Can you work these out from the model? Positions are in its coordinate system, mm. A direction names the side the tool comes from. Coordinates: 2 decimals unless noted, no trailing zeros. Order: outer loops, then holes, each group sorted by start corner. A loop starts at its lowest first (then second) coordinate and runs counter-clockwise, first axis right, second up. Notation, with made-up numbers: (85, -17.5) - (106, -17.5) arc R22 ccw to (106, 15.5) - close; hole circle Ø3 at (27.25, 15). An arc over 180 degrees is marked (long way). Use a Markdown table: item, result. Add a question column.
(1) If I drill on L1, parallel to Y at x = 0, z = -7; L2, parallel to X at y = 1.15, z = -2.25; L3, parallel to X at y = 0, z = -7.3, over which ranges is the centre line in solid material (lowest first)? Write a range as [from, to].
(2) For pin 1 Ø1 at (x, y) = (-2.5, -0.5) entering from +Z; pin 2 Ø2 at (x, z) = (-2.5, -2) entering from +Y; pin 3 Ø1.6 at (x, y) = (-12.5, 0) entering from +Z; pin 4 Ø2.5 at (x, y) = (12, 0) entering from -Z, each with a flat end and sliding along its axis, tell me the tip position at first contact or that it passes through.
(3) I want a section at D-D (x = -8). List the corners of the cut face in (y, z) for me.
(4) I want a section at C-C (z = -7). List the corners of the cut face in (x, y) for me.
(5) I want a section at A-A (x = 12.5). List the corners of the cut face in (y, z) for me.
(6) We'd pull the mould along Z, two halves only. Please class faces 3 (the flat face through (-13, 0, -2)), 4 (the conical face through (-11.082, -0.588, -0.396)), 5 (the conical face through (13.918, -0.588, -0.396)), 6 (the flat face through (15, 0, -1)): pulls with the +Z half, pulls with the -Z half, needs draft (parallel to the pull), parting line crosses it, or undercut.
(7) On a 3-axis mill with a long thin cutter (end or side, diameter ignored), from which of +Z, -Z, +X, -X, +Y, -Y can I reach the whole of each face in a straight line? I mean faces 1 (the flat face through (12, 0, -2)), 2 (the flat face through (-10, 0, 0)). Say none if no direction works.
(8) I want a section at B-B (z = -4.25). List the corners of the cut face in (x, y) for me.
```python
from build123d import *

# Parameters (mm, degrees)
F1_DEPTH = 2.5
F3_R     = 1.5
F4_DEPTH = 1
F4_TAPER = -5
F5_DEPTH = 25


with BuildPart() as f1:
    # F0 (on Front) → F1 (new body, symmetric)
    with BuildSketch(Plane.XZ):
        with BuildLine():
            ThreePointArc((0, -5), (-3.5355339059, -3.5355339059), (-5, 0))
            Line((-5, 0), (-15, 0))
            Line((-15, 0), (-15, -2))
            Line((-15, -2), (-10, -2))
            Line((-10, -2), (-5, -10.6602540378))
            Line((-5, -10.6602540378), (0, -10.6602540378))
            Line((0, -10.6602540378), (5, -10.6602540378))
            Line((5, -10.6602540378), (10, -2))
            Line((10, -2), (15, -2))
            Line((15, -2), (15, 0))
            Line((15, 0), (5, 0))
            ThreePointArc((5, 0), (3.5355339059, -3.5355339059), (0, -5))
        make_face()
    extrude(amount=F1_DEPTH, both=True)

    # F3 (on offset) → F4 (cut)
    with BuildSketch(Plane.XY):
        with Locations((-12.5, 0)):
            Circle(F3_R)
        with Locations((12.5, 0)):
            Circle(F3_R)
    extrude(amount=-F4_DEPTH, taper=F4_TAPER, mode=Mode.SUBTRACT)

    # F3 (on offset) → F5 (cut)
    with BuildSketch(Plane.XY):
        Circle(F3_R)
    extrude(amount=-F5_DEPTH, mode=Mode.SUBTRACT)


solid = f1.part
```
Answers follow:
| question | item | result |
|---|---|---|
| 1 | L1 | y = [-2.5, -1.5], [1.5, 2.5] |
| 1 | L2 | x = [-9.86, -4.47], [4.47, 9.86] |
| 1 | L3 | x = [-6.94, -1.5], [1.5, 6.94] |
| 2 | pin 1 | stops at z = -4 |
| 2 | pin 2 | passes through |
| 2 | pin 3 | stops at z = -1 |
| 2 | pin 4 | stops at z = -2 |
| 3 | outline | (-2.5, -5.46) - (2.5, -5.46) - (2.5, 0) - (-2.5, 0) - close |
| 4 | outline | (-7.11, -2.5) - (7.11, -2.5) - (7.11, 2.5) - (-7.11, 2.5) - close; hole circle Ø3 at (0, 0) |
| 5 | outline | (-2.5, -2) - (2.5, -2) - (2.5, 0) - (1.5, 0) - (1.59, -1) - (-1.59, -1) - (-1.5, 0) - (-2.5, 0) - close |
| 6 | face 3 | pulls with the -Z half |
| 6 | face 4 | undercut |
| 6 | face 5 | undercut |
| 6 | face 6 | needs draft |
| 7 | face 1 | -Z, +X, +Y, -Y |
| 7 | face 2 | +Z, +X, -X, +Y, -Y |
| 8 | outline | (-8.7, -2.5) - (-2.63, -2.5) - (-2.63, 2.5) - (-8.7, 2.5) - close; (2.63, -2.5) - (8.7, -2.5) - (8.7, 2.5) - (2.63, 2.5) - close |
